Solid Edge part; units mm, degrees
sketch "Sketch1" plane through (0, 0, 0) normal (0, -1, 0) x (1, 0, 0)
  line L0 (4, 8) -> (1.5, 8)
  line L1 (1.5, 8) -> (1.5, 11)
  line L2 (1.5, 11) -> (0, 11)
  line L3 (0, 11) -> (0, -11)
  line L4 (0, -11) -> (1.5, -11)
  line L5 (1.5, -11) -> (1.5, -8)
  line L6 (1.5, -8) -> (4, -8)
  line L7 (4, -8) -> (4, -7.5)
  line L8 (4, -7.5) -> (4.8, -7.5)
  line L9 (4.8, -7.5) -> (4.8, 7.5)
  line L10 (4.8, 7.5) -> (4, 7.5)
  line L11 (4, 7.5) -> (4, 8)
revolve "RevolvedProtrusion1" add sketch "Sketch1" angle 360 about axis through (0, 0, 11) along (0, 0, -1)
chamfer "Chaflán_2" distance 0.2 angle 45 4 edges at (-1.5, 0, -11) (-1.5, 0, 11) (-4, 0, 8) (-4, 0, -8)
chamfer "Chaflán_3" distance 1 angle 45 2 edges at (-4.8, 0, -7.5) (-4.8, 0, 7.5)
chamfer "Chamfer1" [suppressed]
Work out the finished part from the listing and answer in its coordinate system (mm). A direction names the side the tool comes from. Give positions to 0.01 mm unless a question says otherwise; leave off trailing zeros. Loops run counter-clockwise (first coordinate to the right, second up) from the corner with the lowest first, then second, coordinate; pieces in that order, holes last. Notation, with made-up numbers: M -2.5,34 L 15.5,34 A29 cw 15.5,70 Z; hole C 24,11.5 d2. An arc over 180 degrees is marked long. One line per item, written item: value. Start each with the question number.
1. Which of the six approach directions +Z, -Z, +X, -X, +Y, -Y give full straight-line access (tool end or side, diameter ignored) to faces 1 (the face through (2, 0, -8)), 2 (the face through (0, 0, 11)), 3 (the face through (2, 0, 8))?
2. Each of these flat-tipped pins is pushed along its axis until it touches: P1, Ø4, axis at x = -3, y = 2.5, coming from the -Z side; P2, Ø3, axis at x = -2.5, z = 2.5, coming from the -Y side; P3, Ø3, axis at x = -0.5, z = -7.5, coming from the -Y side. Where does it stop, or does it pass through?
3. Find section A-A (y = 0). Give the vertices of the cut face in (x, z).
4. Find the intervals of material crossed by probe 1 along Z at (x, y) = (2, 1.75); probe 2 along Z at (x, y) = (-0.75, -4); probe 3 along Y at (x, z) = (3.25, 7), in increasing order.
5. Find section C-C (z = 2.75). Give the vertices of the cut face in (x, y), and give its area (3 significant figures).
Reported:
1. face 1: -Z
1. face 2: +Z, +X, -X, +Y, -Y
1. face 3: +Z
2. P1: stops at z = -8
2. P2: stops at y = -4.69
2. P3: stops at y = -4.8
3. outline: M -4.8,-6.5 L -4,-7.3 L -4,-7.8 L -3.8,-8 L -1.5,-8 L -1.5,-10.8 L -1.3,-11 L 1.3,-11 L 1.5,-10.8 L 1.5,-8 L 3.8,-8 L 4,-7.8 L 4,-7.3 L 4.8,-6.5 L 4.8,6.5 L 4,7.3 L 4,7.8 L 3.8,8 L 1.5,8 L 1.5,10.8 L 1.3,11 L -1.3,11 L -1.5,10.8 L -1.5,8 L -3.8,8 L -4,7.8 L -4,7.3 L -4.8,6.5 Z
4. probe 1: z = -8 to 8
4. probe 2: z = -7.23 to 7.23
4. probe 3: y = -2.82 to 2.82
5. outline: C 0,0 d9.6
5. area: 72.4 mm²
